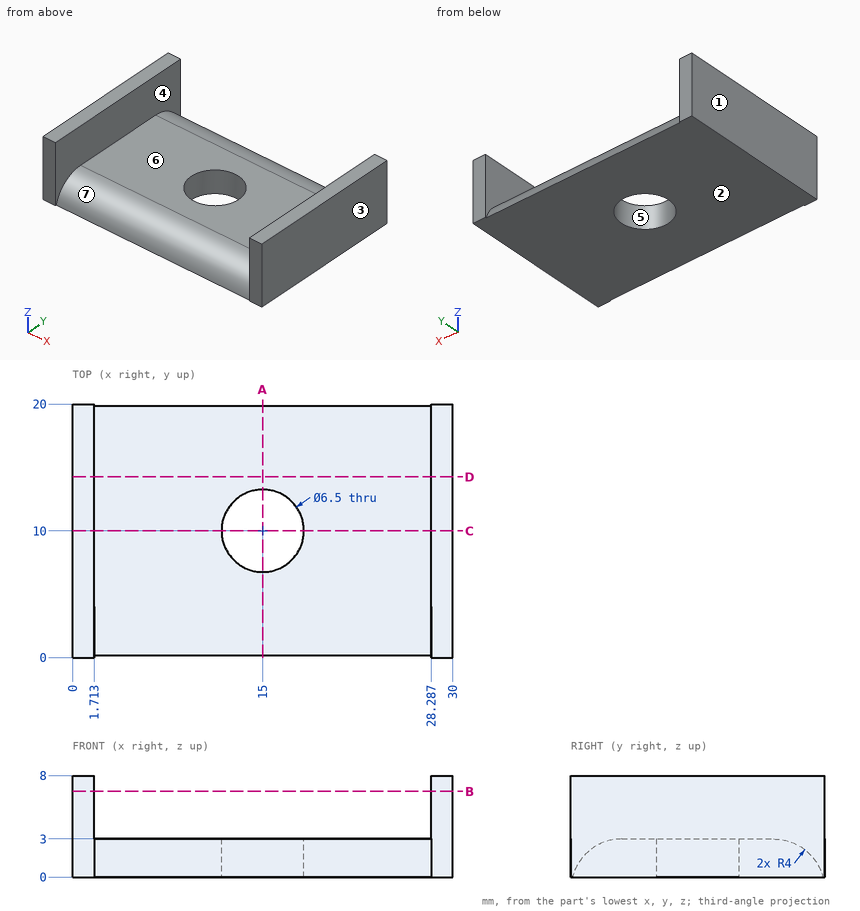
Part print with two shaded views. Sizes in mm from the minimum x, y, z corner. A direction names the side the tool comes from. Round coordinates to 2 decimals unless told otherwise and drop trailing zeros. Order: outer loops, then holes, each group sorted by start corner. A loop starts at its lowest first (then second) coordinate and runs counter-clockwise, first axis right, second up. Notation, with made-up numbers: (-33.75, 17) -> (12.25, 17) arc R17 cw to (12.25, 21) -> close; hole circle Ø1 at (-5.75, -6). An arc over 180 degrees is marked (long way). One line per question, with ' | ' between items.
Q1. Slice it at B-B (z = 6.75). Write the cut outline in (x, y), then the cut area to 3 significant figures.
Completed:
outline: (0, 0) -> (1.71, 0) -> (1.71, 20) -> (0, 20) -> close; (28.29, 0) -> (30, 0) -> (30, 20) -> (28.29, 20) -> close | area: 68.5 mm^2
Q2. Which spindle directions (+Z, -Z, +X, -X, +Y, -Y) get a long thin tool onto all of the face, cutting with end or side? Do the marked faces 5, 6 and 7. Say none if no direction does.
Completed:
face 5: +Z, -Z | face 6: +Z, +Y, -Y | face 7: +Z, -Y
Q3. Slice it at A-A (x = 15). Write the cut outline in (y, z), then the cut area to 3 significant figures.
Completed:
outline: (0.13, 0) -> (6.75, 0) -> (6.75, 3) -> (4, 3) arc R4 ccw to start; (13.25, 0) -> (19.87, 0) arc R4 ccw to (16, 3) -> (13.25, 3) -> close | area: 33.7 mm^2
Q4. Drop flat-ended pins along their axis: pin 1 (2 mm diameter, centred on x = 25, z = 4.5, fed in from +Y); pin 2 (4 mm diameter, centred on x = 12.5, z = 4.5, fed in from -Y); pin 3 (4 mm diameter, centred on x = 25.5, y = 17.5, fed in from +Z). Give the stop position or say it passes through.
Completed:
pin 1: passes through | pin 2: stops at y = 2.06 | pin 3: stops at z = 3
Q5. Slice it at D-D (y = 14.25). Write the cut outline in (x, z), then the cut area to 3 significant figures.
Completed:
outline: (0, 0) -> (30, 0) -> (30, 8) -> (28.29, 8) -> (28.29, 3) -> (1.71, 3) -> (1.71, 8) -> (0, 8) -> close | area: 107 mm^2
Q6. Two-plate mould, pull along X, no slides. Class the marked faces 1, 2, 3 and 4: released by +X, released by -X, zero draft, split by the parting line, or undercut.
Completed:
face 1: released by -X | face 2: zero draft | face 3: released by +X | face 4: undercut
Q7. Probe probe 1 along X at (y, z) = (11.5, 5.5); probe 2 along Z at (x, y) = (17, 12.75); probe 3 along Y at (x, z) = (15, 2.1). List the from-to ranges inside material, lowest first.
Completed:
probe 1: x = 0 to 1.71, 28.29 to 30 | probe 2: z = 0 to 3 | probe 3: y = 1.47 to 6.75, 13.25 to 18.53
Q8. Slice it at C-C (y = 10). Write the cut outline in (x, z).
Completed:
outline: (0, 0) -> (11.75, 0) -> (11.75, 3) -> (1.71, 3) -> (1.71, 8) -> (0, 8) -> close; (18.25, 0) -> (30, 0) -> (30, 8) -> (28.29, 8) -> (28.29, 3) -> (18.25, 3) -> close
